```python
from build123d import *

# Parameters (mm, degrees)
BOSS_EXTRUDE1_DEPTH = 100
FILLET1_R           = 5
SKETCH2_R           = 5
CUT_EXTRUDE1_DEPTH  = 75
SKETCH3_W           = 40
SKETCH3_H           = 13
BOSS_EXTRUDE2_DEPTH = 12.5
SKETCH9_R           = 7.5
BOSS_EXTRUDE6_DEPTH = 15
SKETCH10_R          = 4
CUT_EXTRUDE3_DEPTH  = 15


with BuildPart() as part:
    # Sketch1 → Boss-Extrude1 (new body)
    with BuildSketch(Plane.XY):
        Polygon((0, 0), (35, 0), (35, -20), (0, -20), (0, -25), (40, -25), (40, 5), (0, 5), align=None)
    extrude(amount=BOSS_EXTRUDE1_DEPTH)

    # Fillet1
    fillet1_edges = [part.edges().sort_by_distance(p)[0] for p in [
        (35, -20, 50),
        (35, 0, 50),
    ]]
    fillet(fillet1_edges, radius=FILLET1_R)

    # Sketch2 → Cut-Extrude1 (cut)
    with BuildSketch(Plane(origin=(0, 5, 0), x_dir=(1, 0, 0), z_dir=(0, 1, 0))):
        with Locations(Location((15, -64, 0), (0, 0, 180))):
            Circle(SKETCH2_R)
        with Locations(Location((15, -36, 0), (0, 0, 270))):
            Circle(SKETCH2_R)
    extrude(amount=-CUT_EXTRUDE1_DEPTH, mode=Mode.SUBTRACT)

    # Sketch3 → Boss-Extrude2 (add)
    with BuildSketch(Plane.XZ.offset(25)):
        with Locations((20, 50)):
            Rectangle(SKETCH3_W, SKETCH3_H)
    extrude(amount=BOSS_EXTRUDE2_DEPTH)

    # Sketch9 → Boss-Extrude6 (add)
    with BuildSketch(Plane(origin=(40, 0, 0), x_dir=(0, 0, -1), z_dir=(1, 0, 0))):
        with Locations(Location((-50, -10, 0), (0, 0, 180))):
            Circle(SKETCH9_R)
    extrude(amount=BOSS_EXTRUDE6_DEPTH)

    # Sketch10 → Cut-Extrude3 (cut)
    with BuildSketch(Plane(origin=(55, 0, 0), x_dir=(0, 0, -1), z_dir=(1, 0, 0))):
        with Locations((-50, -10)):
            Circle(SKETCH10_R)
    extrude(amount=-CUT_EXTRUDE3_DEPTH, mode=Mode.SUBTRACT)


solid = part.part
```
CAD build for the part. Positions are in the model's coordinates, mm. A direction names the side the tool comes from. Coordinates: 2 decimals unless noted, no trailing zeros. Order: outer loops, then holes, each group sorted by start corner. A loop starts at its lowest first (then second) coordinate and runs counter-clockwise, first axis right, second up. Notation, with made-up numbers: M 77,-19 L 136,-19 A5 ccw 136,-13 Z; hole C -31.75,-19.5 d1. An arc over 180 degrees is marked long. Answer as CSV lines item,"result".
1) Cut at B-B (x = 25.5). List the corners of the cut face in (y, z), then the cut area to 3 significant figures.
Verdict:
outline,"M -37.5,43.5 L -25,43.5 L -25,0 L -20,0 L -20,100 L -25,100 L -25,56.5 L -37.5,56.5 Z; M 0,0 L 5,0 L 5,100 L 0,100 Z"
area,"1,160 mm2"
2) 3-axis set-ups, long thin cutter, end or side, ignore diameter. For faces 1 (the flat face through (20, -25, 78)), 2 (the cylindrical face through (47.6, -12.4, 53.2)), 3 (the flat face through (20, -25, 21)), 4 (the cylindrical face through (34, -18, 51)): which of +Z, -Z, +X, -X, +Y, -Y reach the whole face in a straight line?
Verdict:
face 1,"+Z, +X, -X, -Y"
face 2,"+X"
face 3,"-Z, +X, -X, -Y"
face 4,"+Z, -Z, -X"
3) Cut at C-C (x = 15). List the corners of the cut face in (y, z).
Verdict:
outline,"M -37.5,43.5 L -25,43.5 L -25,41 L -20,41 L -20,59 L -25,59 L -25,56.5 L -37.5,56.5 Z; M -25,0 L -20,0 L -20,31 L -25,31 Z; M -25,69 L -20,69 L -20,100 L -25,100 Z; M 0,0 L 5,0 L 5,31 L 0,31 Z; M 0,41 L 5,41 L 5,59 L 0,59 Z; M 0,69 L 5,69 L 5,100 L 0,100 Z"
4) Mould opens along Z. For faces 5 (the cylindrical face through (12, 3, 32)), 6 (the flat face through (24.2, 0.2, 0)), 7 (the flat face through (20, -37.5, 50)) say: released by +Z, released by -Z, zero draft, split by the parting line, or undercut.
Verdict:
face 5,"undercut"
face 6,"released by -Z"
face 7,"zero draft"
5) Drill centre lines: L1, parallel to X at y = 3, z = 36; L2, parallel to Y at x = 51, z = 50; L3, parallel to Y at x = 18.5, z = 26.5. Where is each one in solid material? Low to high. Write a range as from..to.
Verdict:
L1,"0..10, 20..40"
L2,"-17.5..-14, -6..-2.5"
L3,"-25..-20, 0..5"
6) Cut at A-A (z = 64). List the corners of the cut face in (x, y).
Verdict:
outline,"M 0,-25 L 10,-25 L 10,-20 L 0,-20 Z; M 0,0 L 10,0 L 10,5 L 0,5 Z; M 20,-25 L 40,-25 L 40,5 L 20,5 L 20,0 L 30,0 A5 cw 35,-5 L 35,-15 A5 cw 30,-20 L 20,-20 Z"
7) Flat gauge pins, fed straight in: P1, Ø4, axis at x = 19.5, y = -33, coming from the +Z side; P2, Ø10, axis at x = 21, z = 12, coming from the -Y side; P3, Ø6, axis at x = 27, y = -32.5, coming from the -Z side. Where does each tip first touch, or does it go through?
Verdict:
P1,"z = 56.5"
P2,"y = -25"
P3,"z = 43.5"
8) Cut at D-D (y = -21). List the corners of the cut face in (x, z).
Verdict:
outline,"M 0,0 L 40,0 L 40,100 L 0,100 Z; hole C 15,36 d10; hole C 15,64 d10"
